Autodesk Inventor part; units mm, degrees
ref_plane "Work Plane1" through (0, 0, 10) normal (0, 0, 1) x (1, 0, 0)
ref_plane "YZ Plane" through (0, 0, 0) normal (1, 0, 0) x (0, 1, 0)
ref_plane "XZ Plane" through (0, 0, 0) normal (0, 1, 0) x (-1, 0, 0)
sketch "Sketch1" plane through (0, 0, 0) normal (0, 0, 1) x (1, 0, 0)
  line L0 (-6, 0) -> (6, 0) construction
  line L1 (-6, -5) -> (6, -5)
  line L2 (6, 5) -> (-6, 5)
  arc A0 (-6, 5) -> (-6, -5) centre (-6, 0) ccw
  arc A1 (6, -5) -> (6, 5) centre (6, 0) ccw
  point P0 (0, 0)
  point P1 (0, 0)
  dimension "d0" = 5
  dimension "d1" = 12
extrude "Extrusion1" add sketch "Sketch1" along normal mid plane 40
sketch "Sketch2" plane through (0, 0, 20) normal (0, 0, 1) x (1, 0, 0)
  arc A0 (-6, 5) -> (-6, -5) centre (-6, 0) ccw
  arc A1 (6, -5) -> (6, 5) centre (6, 0) ccw
  point P0 (0, 0)
hole "Hole1" at (-6, 0, 20) at (6, 0, 20) direction (0, 0, -1) diameter 3.2 end through all
ref_plane "Work Plane1" through (0, 0, 10) normal (0, 0, 1) x (1, 0, 0)
sketch "Sketch3" plane through (0, 0, 10) normal (0, 0, 1) x (1, 0, 0)
  circle A0 centre (-6, 0) radius 1.6
  line L0 (-7.5877, 2.75) -> (-4.4123, 2.75)
  line L1 (-4.4123, 2.75) -> (-2.8246, 0)
  line L2 (-2.8246, 0) -> (-4.4123, -2.75)
  line L3 (-4.4123, -2.75) -> (-7.5877, -2.75)
  line L4 (-7.5877, -2.75) -> (-9.1754, 0)
  line L5 (-9.1754, 0) -> (-7.5877, 2.75)
  line L6 (-7.5877, 2.75) -> (-10.1758, 2.75)
  arc A1 (-6, 5) -> (-6, -5) centre (-6, 0) ccw
  line L7 (-7.5877, -2.75) -> (-10.1758, -2.75)
  point P0 (0, 0)
  dimension "d12" = 5.5
extrude "Extrusion2" cut sketch "Sketch3" against normal blind 4
mirror "Mirror1" about plane through (0, 0, 0) normal (1, 0, 0) of "Extrusion2"
mirror "Mirror2" about plane through (0, 0, 0) normal (0, 0, 1) of "Extrusion2", "Mirror1"
properties part number "Standoff" material "ABS Plastic"
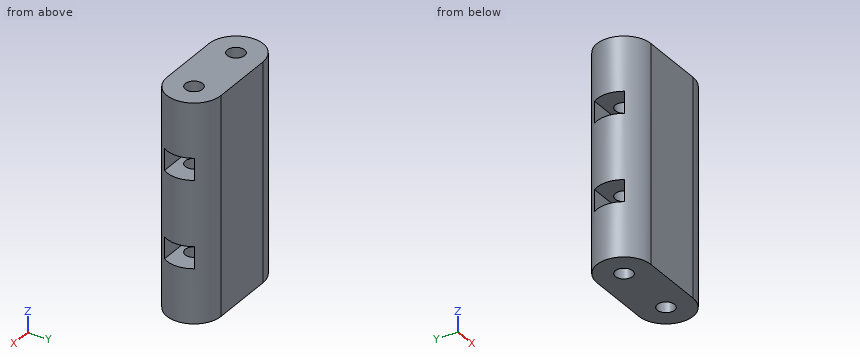
Geometry check sheet. Reference: the model listing, model coordinates, mm. Give positions to 0.01 mm unless a question says otherwise; leave off trailing zeros. Write each loop counter-clockwise with the first axis right and the second up, starting at its lowest first coordinate (ties: lowest second). Pieces come first, ordered by that corner, then holes.
1) Thickness scan on line 1 (X direction, y = 0, z = 18.25); line 2 (X direction, y = 1, z = -11.5); line 3 (Y direction, x = 6, z = -12). Record the ranges inside material, lowest first.
Values follow:
line 1: x = -11 to -7.6, -4.4 to 4.4, 7.6 to 11
line 2: x = -10.9 to -7.25, -4.75 to 4.75, 7.25 to 10.9
line 3: y = -5 to -1.6, 1.6 to 5
2) Cross-section at B-B (x = -8.5). Record the boundary of the cut face in (y, z).
Values follow:
outline: (-4.33, -20) - (4.33, -20) - (4.33, 20) - (-4.33, 20) - close; hole (-2.75, -10) - (2.75, -10) - (2.75, -6) - (-2.75, -6) - close; hole (-2.75, 6) - (2.75, 6) - (2.75, 10) - (-2.75, 10) - close
3) Cross-section at D-D (x = 5.5). Record the boundary of the cut face in (y, z).
Values follow:
outline: (-5, -20) - (-1.52, -20) - (-1.52, -10) - (-2.75, -10) - (-2.75, -6) - (-1.52, -6) - (-1.52, 6) - (-2.75, 6) - (-2.75, 10) - (-1.52, 10) - (-1.52, 20) - (-5, 20) - close; (1.52, -20) - (5, -20) - (5, 20) - (1.52, 20) - (1.52, 10) - (2.75, 10) - (2.75, 6) - (1.52, 6) - (1.52, -6) - (2.75, -6) - (2.75, -10) - (1.52, -10) - close
4) Cross-section at A-A (z = 3). Record the boundary of the cut face in (x, y).
Values follow:
outline: (-6, -5) - (6, -5) arc R5 ccw to (6, 5) - (-6, 5) arc R5 ccw to start; hole circle Ø3.2 at (-6, 0); hole circle Ø3.2 at (6, 0)
5) Cross-section at C-C (y = -2.25). Record the boundary of the cut face in (x, z).
Values follow:
outline: (-10.47, -20) - (10.47, -20) - (10.47, -10) - (4.12, -10) - (4.12, -6) - (10.47, -6) - (10.47, 6) - (4.12, 6) - (4.12, 10) - (10.47, 10) - (10.47, 20) - (-10.47, 20) - (-10.47, 10) - (-4.12, 10) - (-4.12, 6) - (-10.47, 6) - (-10.47, -6) - (-4.12, -6) - (-4.12, -10) - (-10.47, -10) - close
6) Go/stop test with flat-tipped pins: pin 1 Ø1.2 at (x, z) = (-8.5, -8) entering from +Y; pin 2 Ø2 at (x, z) = (-8, 8.5) entering from -Y; pin 3 Ø1 at (y, z) = (-2.5, -5.5) entering from +X. Record where each tip stops, or that it passes through.
Values follow:
pin 1: stops at y = 4.62
pin 2: stops at y = -4.9
pin 3: stops at x = 10.58
